Check sheet for the drawn part. Datum: minimum x, y, z corner. Units: mm. A direction names the side the tool comes from. Coordinates: 2 decimals unless noted, no trailing zeros. Write each loop counter-clockwise with the first axis right and the second up, starting at its lowest first coordinate (ties: lowest second). Pieces come first, ordered by that corner, then holes. Notation, with made-up numbers: (-21, 47.5) -> (18, 47.5) arc R35 ccw to (18, 85.5) -> close; hole circle Ø10 at (-16, -39). An arc over 180 degrees is marked (long way). Answer in a Markdown table with one row per item. Add a question column.
Q1. Tool access check on the marked faces 1 and 2. Record the directions out of +Z, -Z, +X, -X, +Y, -Y that give a thin tool (end or side, any length) a straight path to the whole face; none if there is none.
Q2. Thickness scan on line 1 (Y direction, x = 20, z = 6) (1 decimal); line 2 (Z direction, x = 101.6, y = 2.3). Record the ranges inside material, lowest first.
Q3. Section check B-B, the plane y = 10.5. Record the boundary of the cut face in (x, z) (1 decimal).
Q4. Gauge pin test, flat ends, axial feed: P1, Ø5, axis at x = 98, y = 20, coming from the +Z side (1 decimal); P2, Ø10, axis at x = 75.5, z = 17, coming from the +Y side (1 decimal); P3, Ø4, axis at y = 10, z = 3.5, coming from the -X side. Record the tip position at first contact, or that the pin passes through.
Q5. Section check A-A, the plane x = 101.6. Record the boundary of the cut face in (y, z) (1 decimal), and give its area (3 significant figures).
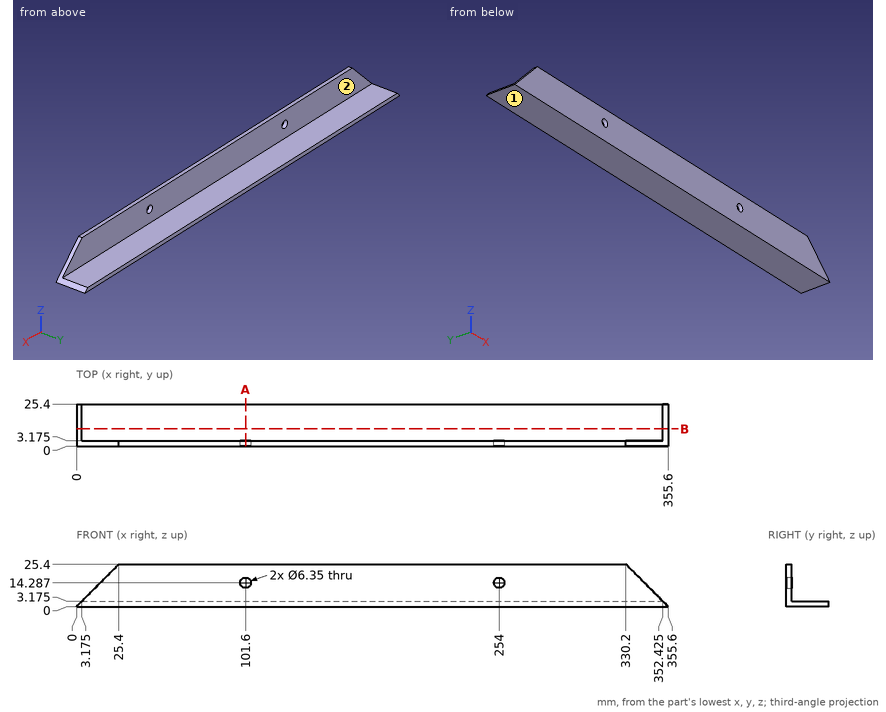
Calculated:
| question | item | result |
|---|---|---|
| 1 | face 1 | -Z, +X, -X, +Y, -Y |
| 1 | face 2 | +Z, +X, -X, +Y |
| 2 | line 1 | y = 0 to 3.2 |
| 2 | line 2 | z = 0 to 11.11, 17.46 to 25.4 |
| 3 | outline | (0, 0) -> (355.6, 0) -> (352.4, 3.2) -> (3.2, 3.2) -> close |
| 4 | P1 | stops at z = 3.2 |
| 4 | P2 | stops at y = 3.2 |
| 4 | P3 | stops at x = 1.5 |
| 5 | outline | (0, 0) -> (25.4, 0) -> (25.4, 3.2) -> (3.2, 3.2) -> (3.2, 11.1) -> (0, 11.1) -> close; (0, 17.5) -> (3.2, 17.5) -> (3.2, 25.4) -> (0, 25.4) -> close |
| 5 | area | 131 mm² |
